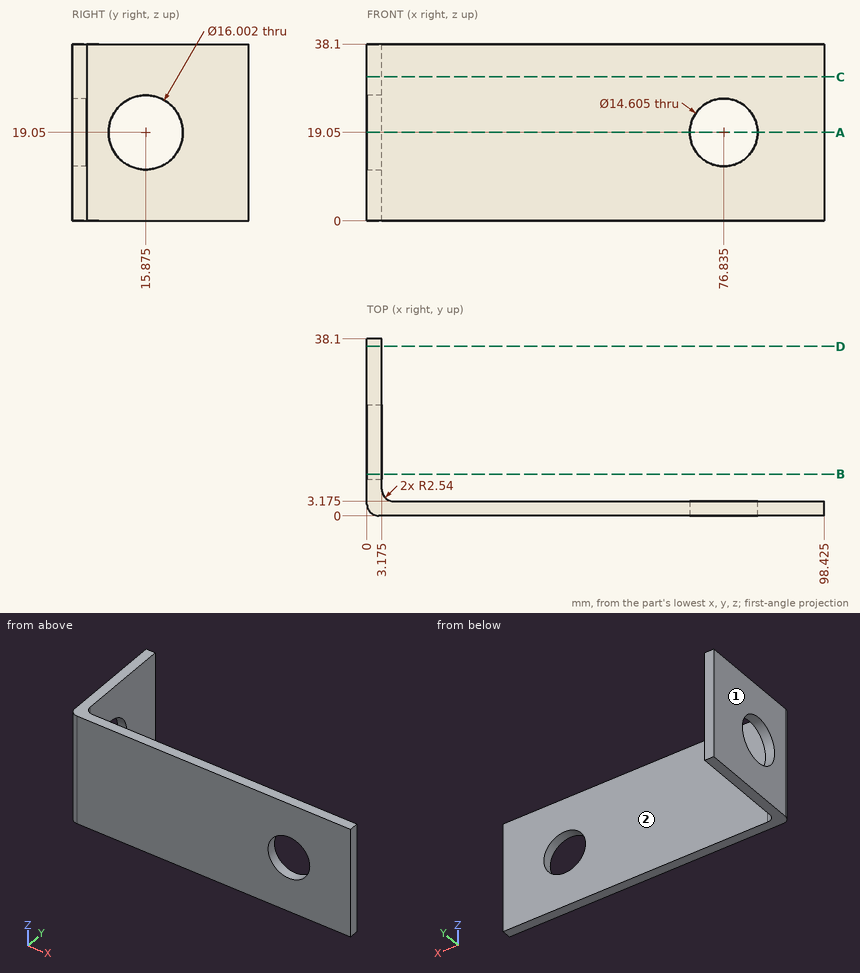
Answer from the drawing. Dimensions are ordinates in mm from the lowest x, y and z of the part. A direction names the side the tool comes from. Round coordinates to 2 decimals unless told otherwise and drop trailing zeros. Write each loop counter-clockwise with the first axis right and the second up, starting at its lowest first coordinate (ties: lowest second). Pieces come first, ordered by that corner, then holes. Notation, with made-up numbers: (-1.75, 56.25) -> (42.25, 56.25) arc R17 ccw to (42.25, 81.25) -> close; hole circle Ø3 at (83, 62.5). An arc over 180 degrees is marked (long way). Write each question's results on one line, items separated by ' | '.
1) The part is cut by section A-A (z = 19.05). Write down the section's boundary in (x, y) (1 decimal), and give its area (3 significant figures).
Findings:
outline: (0, 2.5) arc R2.5 ccw to (2.5, 0) -> (69.5, 0) -> (69.5, 3.2) -> (5.7, 3.2) arc R2.5 cw to (3.2, 5.7) -> (3.2, 7.9) -> (0, 7.9) -> close; (0, 23.9) -> (3.2, 23.9) -> (3.2, 38.1) -> (0, 38.1) -> close; (84.1, 0) -> (98.4, 0) -> (98.4, 3.2) -> (84.1, 3.2) -> close | area: 326 mm²
2) The part is cut by section C-C (z = 31). Write down the section's boundary in (x, y) (3 decimals), and give its area (3 significant figures).
Findings:
outline: (0, 2.54) arc R2.54 ccw to (2.54, 0) -> (98.425, 0) -> (98.425, 3.175) -> (5.715, 3.175) arc R2.54 cw to (3.175, 5.715) -> (3.175, 38.1) -> (0, 38.1) -> close | area: 423 mm²
3) The part is cut by section B-B (y = 9). Write down the section's boundary in (x, z) (3 decimals).
Findings:
outline: (0, 0) -> (3.175, 0) -> (3.175, 14.957) -> (0, 14.957) -> close; (0, 23.143) -> (3.175, 23.143) -> (3.175, 38.1) -> (0, 38.1) -> close
4) Consider line 1 along Y through (x, z) = (2.55, 19.05); line 2 along X through (y, z) = (25.5, 35) (3 decimals); line 3 along Y through (x, z) = (1.1, 19.05). Determine where each line is inside the solid, lowest interval first. Write a range as [from, to].
Findings:
line 1: y = [0, 7.87], [23.88, 38.1] | line 2: x = [0, 3.175] | line 3: y = [0.45, 7.87], [23.88, 38.1]
5) The part is cut by section D-D (y = 36.5). Write down the section's boundary in (x, z) (3 decimals).
Findings:
outline: (0, 0) -> (3.175, 0) -> (3.175, 38.1) -> (0, 38.1) -> close
6) Flat-ended cylindrical pins translate along their axes: pin 1 (4 mm diameter, centred on x = 21.5, z = 26.5, fed in from +Y) (3 decimals); pin 2 (9 mm diameter, centred on x = 76.835, z = 19.05, fed in from +Y); pin 3 (16 mm diameter, centred on y = 27.5, z = 17.5, fed in from +X) (3 decimals). Find the tip coordinate at first contact, or state that the pin passes through.
Findings:
pin 1: stops at y = 3.175 | pin 2: passes through | pin 3: stops at x = 3.175
7) Which of the six approach directions +Z, -Z, +X, -X, +Y, -Y give full straight-line access (tool end or side, diameter ignored) to the marked faces 1 and 2?
Findings:
face 1: +Z, -Z, -X, +Y, -Y | face 2: +Z, -Z, +X, +Y
